Work out the finished part from the listing and answer in its coordinate system (mm). Give positions to 0.01 mm unless a question says otherwise; leave off trailing zeros. Order: outer loops, then holes, each group sorted by start corner. A loop starts at its lowest first (then second) coordinate and runs counter-clockwise, first axis right, second up. Notation, with made-up numbers: (5.25, 82.5) - (41.25, 82.5) arc R34 ccw to (41.25, 118.5) - close; hole circle Ø3 at (85, 63). An arc over 180 degrees is marked (long way). Return JSON: item names as keys, results as strings. Group by question number.
Autodesk Inventor part; units mm, degrees
ref_plane "YZ Plane" through (0, 0, 0) normal (1, 0, 0) x (0, 1, 0)
ref_plane "XZ Plane" through (0, 0, 0) normal (0, 1, 0) x (-1, 0, 0)
ref_plane "XY Plane" through (0, 0, 0) normal (0, 0, 1) x (1, 0, 0)
sketch "Sketch1" plane through (0, 0, 0) normal (0, 0, 1) x (1, 0, 0)
  circle A0 centre (0, 0) radius 43.0276
  circle A1 centre (83.6836, -4.7804) radius 12.4968
  circle A2 centre (0, 0) radius 44.0436
  circle A3 centre (83.6836, -4.7804) radius 13.5128
  line L0 (13.6771, -41.8662) -> (87.8798, -17.6251)
  line L1 (13.3616, -40.9004) -> (87.5643, -16.6593)
  line L2 (88.8918, 6.5794) -> (17.9323, 39.1127)
  line L3 (89.3152, 7.503) -> (18.3557, 40.0363)
  point P0 (17.6469, -33.9959)
  point P1 (17.4567, 34.094)
  dimension "d0" = 86.0552
  dimension "d1" = 24.9936
  dimension "d2" = 83.82
  dimension "d3" = 88.0872
  dimension "d4" = 27.0256
  dimension "d5" = 1.016
  dimension "d6" = 1.016
extrude "Extrusion1" add sketch "Sketch1" along normal blind 9.0932 contours A0 L1 A2 L2 | A2 L3 A3 L2 | L1 A3 L0 A2 | A3 L1 A1 L2 picked at (-23.5196, -36.5948) picked at (90.0516, 6.6643)
properties part number "Diff Motor Belts"
1. Each of these flat-tipped pins is pushed along its axis until it touches: pin 1 (1.5 mm diameter, centred on y = 0, z = 5.5, fed in from +X); pin 2 (4 mm diameter, centred on y = 19, z = 5, fed in from +X); pin 3 (2 mm diameter, centred on y = 20.5, z = 6, fed in from -X). Where does it stop, or does it pass through?
2. The part is cut by section C-C (z = 7.25). Give the vertices of the cut face in (x, y), and give its area (3 significant figures).
3. The part is cut by section B-B (y = 0). Give the vertices of the cut face in (x, z).
4. The part is cut by section A-A (x = 0). Give the vertices of the cut face in (y, z).
5. Consider probe 1 along Y at (x, z) = (0, 6); probe 2 along Y at (x, z) = (32, 7); probe 3 along X at (y, z) = (0, 4.25). Determine where each line is inside the solid, lowest interval first. Write a range as from..to.
6. Determine the mould class of faces 1 (the cylindrical face through (-44.024, 1.315, 4.483)), 2 (the flat face through (54.332, 23.542, 4.483)), 3 (the cylindrical face through (-43.01, 1.28, 4.48)), 4 (the flat face through (50, -30, 4)) for opening direction Y: released by +Y, released by -Y, zero draft, split by the parting line, or undercut.
Answers:
{
 "1": {"pin 1": "stops at x = 96.58", "pin 2": "stops at x = 68.6", "pin 3": "stops at x = -39.49"},
 "2": {"outline": "(13.68, -41.87) - (87.88, -17.63) arc R13.51 ccw to (89.32, 7.5) - (18.36, 40.04) arc R44.04 ccw (long way) to start; hole (13.36, -40.9) - (87.56, -16.66) arc R12.5 ccw to (88.89, 6.58) - (17.93, 39.11) arc R43.03 ccw (long way) to start", "area": "362 mm^2"},
 "3": {"outline": "(-44.04, 0) - (-43.03, 0) - (-43.03, 9.09) - (-44.04, 9.09) - close; (95.23, 0) - (96.32, 0) - (96.32, 9.09) - (95.23, 9.09) - close"},
 "4": {"outline": "(-44.04, 0) - (-43.03, 0) - (-43.03, 9.09) - (-44.04, 9.09) - close; (43.03, 0) - (44.04, 0) - (44.04, 9.09) - (43.03, 9.09) - close"},
 "5": {"probe 1": "y = -44.04..-43.03, 43.03..44.04", "probe 2": "y = -35.88..-34.81, 32.66..33.78", "probe 3": "x = -44.04..-43.03, 95.23..96.32"},
 "6": {"face 1": "split by the parting line", "face 2": "released by +Y", "face 3": "undercut", "face 4": "released by -Y"}
}
